Print and shaded views of the part. All mm, measured from the part's lowest x, y and z. A direction names the side the tool comes from. Round coordinates to 2 decimals unless told otherwise and drop trailing zeros. Loops run counter-clockwise (first coordinate to the right, second up) from the corner with the lowest first, then second, coordinate; pieces in that order, holes last. Notation, with made-up numbers: (-12.75, 15) - (30.25, 15) arc R21 cw to (30.25, 30) - close; hole circle Ø10 at (51, 43.25). An arc over 180 degrees is marked (long way). Answer as a JSON object with one key per item and string values.
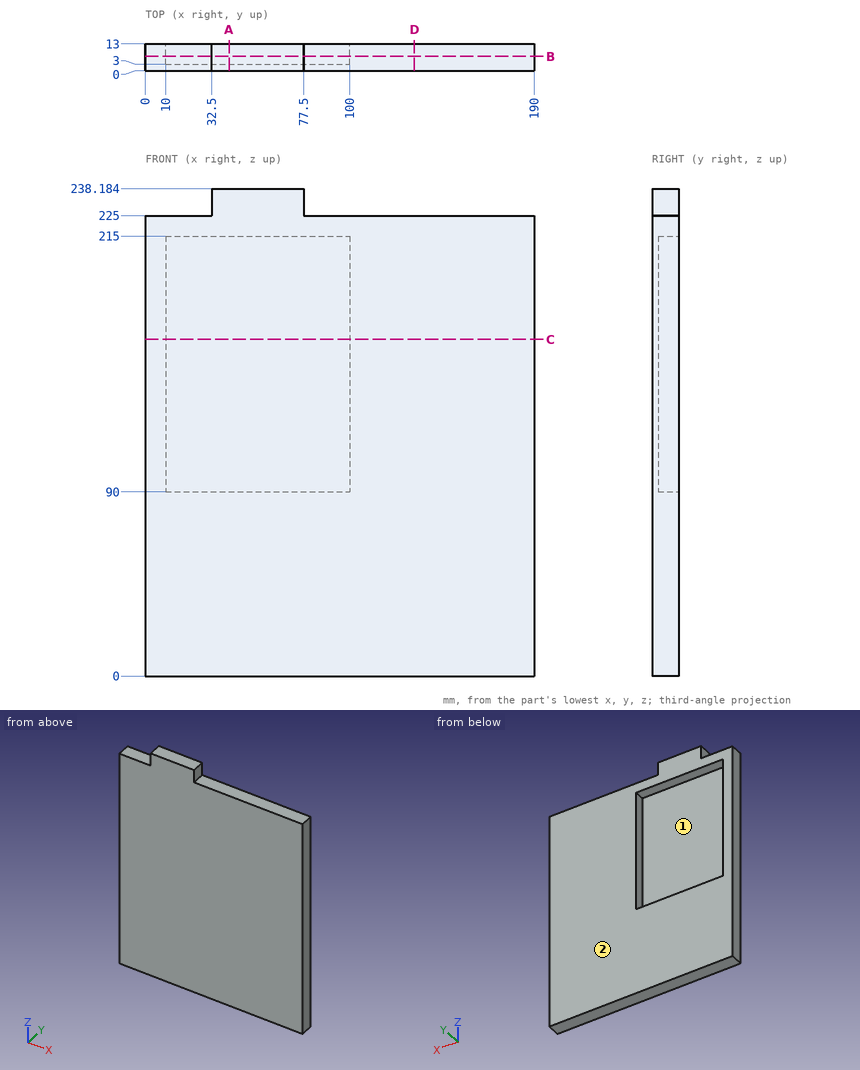
1) Slice it at D-D on x = 131.5. List the corners of the cut face in (y, z), then the cut area to 4 significant figures.
Values follow:
{"outline": "(0, 0) - (13, 0) - (13, 225) - (0, 225) - close", "area": "2,925 mm²"}
2) Drop flat-ended pins along their axis: P1, Ø4, axis at y = 8, z = 229.5, coming from the -X side; P2, Ø6, axis at x = 46, z = 181, coming from the +Y side; P3, Ø4, axis at y = 5.5, z = 231, coming from the +X side. Give the stop position or say it passes through.
Values follow:
{"P1": "x = 32.5", "P2": "y = 3", "P3": "x = 77.5"}
3) Slice it at B-B on y = 7. List the corners of the cut face in (x, z), then the cut area to 3 significant figures.
Values follow:
{"outline": "(0, 0) - (190, 0) - (190, 225) - (77.5, 225) - (77.5, 238.18) - (32.5, 238.18) - (32.5, 225) - (0, 225) - close; hole (10, 90) - (100, 90) - (100, 215) - (10, 215) - close", "area": "32,100 mm²"}
4) Tool access for the marked faces 1 and 2: list every direction of +Z, -Z, +X, -X, +Y, -Y with a clear straight run to the whole face (end or side of a thin tool).
Values follow:
{"face 1": "+Y", "face 2": "+Z, -Z, +X, -X, +Y"}
5) Slice it at C-C on z = 164.5. List the corners of the cut face in (x, y).
Values follow:
{"outline": "(0, 0) - (190, 0) - (190, 13) - (100, 13) - (100, 3) - (10, 3) - (10, 13) - (0, 13) - close"}
6) Probe probe 1 along Z at (x, y) = (31, 9.5); probe 2 along X at (y, z) = (11.5, 184); probe 3 along Z at (x, y) = (58.5, 9.75). List the from-to ranges inside material, lowest first.
Values follow:
{"probe 1": "0 to 90, 215 to 225", "probe 2": "0 to 10, 100 to 190", "probe 3": "0 to 90, 215 to 238.18"}
7) Slice it at A-A on x = 41. List the corners of the cut face in (y, z).
Values follow:
{"outline": "(0, 0) - (13, 0) - (13, 90) - (3, 90) - (3, 215) - (13, 215) - (13, 238.18) - (0, 238.18) - close"}
